Design review of the part built by this model. Coordinates are the model's own, in mm. A direction names the side the tool comes from. Give positions to 0.01 mm unless a question says otherwise; leave off trailing zeros. Write each loop counter-clockwise with the first axis right and the second up, starting at its lowest first coordinate (ties: lowest second). Pieces come first, ordered by that corner, then holes. Notation, with made-up numbers: (53.5, 66) - (108.5, 66) arc R17 ccw to (108.5, 73) - close; hole circle Ø5 at (87, 9). An arc over 180 degrees is marked (long way). Use a Markdown table: item, result. Add a question column.
```python
from build123d import *

# Parameters (mm, degrees)
BASE_DEPTH                = 38.1
DOVETAIL_CUTS_DEPTH       = 30.48
SKETCH3_R                 = 31.115
LOWER_WASHER_LIP_DEPTH    = 0.8128
SKETCH4_R                 = 44.069
SKETCH4_R_2               = 41.529
RETAINING_LIP_DEPTH       = 1.8288
SKETCH6_R                 = 30.48
UPPER_BEARING_LIP_DEPTH   = 2.797175
SKETCH7_R                 = 22.225
CENTRAL_SHAFT_DEPTH       = 26.67
SKETCH5_R                 = 7.62
NUT_CLEARANCE_SHAFT_DEPTH = 44.45
SKETCH8_R                 = 10.795
THROUGH_SHAFT_DEPTH       = 14.7574
SKETCH9_R                 = 4.1275
THROUGH_HOLE_DEPTH        = 108.091797456
NUT_SLOT_DEPTH            = 5.6007
UPPER_START               = -1.016
SKETCH11_R                = 10.795
SKETCH11_R_2              = 9.398
UPPER_WASHER_LIP_DEPTH    = 1.016
FILLET2_R                 = 50.8


with BuildPart() as part:
    # Sketch1 → Base (new body)
    with BuildSketch(Plane(origin=(0, 0, 0), x_dir=(1, 0, 0), z_dir=(0, 1, 0))):
        Polygon((-47.732745366, -19.7715505), (-47.732745366, 19.7715505), (-31.058071097, 31.058071097), (-19.7715505, 47.732745366), (19.7715505, 47.732745366), (31.058071097, 31.058071097), (47.732745366, 19.7715505), (47.732745366, -19.7715505), (31.058071097, -31.058071097), (19.7715505, -47.732745366), (-19.7715505, -47.732745366), (-31.058071097, -31.058071097), align=None)
    extrude(amount=BASE_DEPTH)

    # Sketch2 → Dovetail cuts (cut)
    with BuildSketch(Plane.XZ):
        Polygon((6.055553628, -47.732745366), (-6.055553628, -47.732745366), (-11.43, -17.252745366), (11.43, -17.252745366), align=None)
        Polygon((-17.252745366, -11.43), (-17.252745366, 11.43), (-47.732745366, 6.055553628), (-47.732745366, -6.055553628), align=None)
        Polygon((17.252745366, 11.43), (17.252745366, -11.43), (47.732745366, -6.055553628), (47.732745366, 6.055553628), align=None)
        Polygon((6.055553628, 47.732745366), (11.43, 17.252745366), (-11.43, 17.252745366), (-6.055553628, 47.732745366), align=None)
    extrude(amount=-DOVETAIL_CUTS_DEPTH, mode=Mode.SUBTRACT)

    # Sketch3 → Lower washer lip (add)
    with BuildSketch(Plane(origin=(0, 38.1, 0), x_dir=(1, 0, 0), z_dir=(0, 1, 0))):
        with Locations(Location((0, 0, 0), (0, 0, 270))):
            Circle(SKETCH3_R)
    extrude(amount=LOWER_WASHER_LIP_DEPTH)

    # Sketch4 → Retaining lip (add)
    with BuildSketch(Plane(origin=(0, 38.1, 0), x_dir=(1, 0, 0), z_dir=(0, 1, 0))):
        with Locations(Location((0, 0, 0), (0, 0, 45.946261879))):
            Circle(SKETCH4_R)
        with Locations(Location((0, 0, 0), (0, 0, 270))):
            Circle(SKETCH4_R_2, mode=Mode.SUBTRACT)
    extrude(amount=RETAINING_LIP_DEPTH)

    # Sketch6 → Upper bearing lip (add)
    with BuildSketch(Plane(origin=(0, 38.9128, 0), x_dir=(1, 0, 0), z_dir=(0, 1, 0))):
        with Locations(Location((0, 0, 0), (0, 0, 270))):
            Circle(SKETCH6_R)
    extrude(amount=UPPER_BEARING_LIP_DEPTH)

    # Sketch7 → Central shaft (add)
    with BuildSketch(Plane(origin=(0, 41.709975, 0), x_dir=(1, 0, 0), z_dir=(0, 1, 0))):
        with Locations(Location((0, 0, 0), (0, 0, 270))):
            Circle(SKETCH7_R)
    extrude(amount=CENTRAL_SHAFT_DEPTH)

    # Sketch5 → Nut clearance shaft (cut)
    with BuildSketch(Plane.XZ):
        with Locations(Location((0, 0, 0), (0, 0, 270))):
            Circle(SKETCH5_R)
    extrude(amount=-NUT_CLEARANCE_SHAFT_DEPTH, mode=Mode.SUBTRACT)

    # Sketch8 → Through Shaft (add)
    with BuildSketch(Plane(origin=(0, 68.379975, 0), x_dir=(1, 0, 0), z_dir=(0, 1, 0))):
        with Locations(Location((0, 0, 0), (0, 0, 90))):
            Circle(SKETCH8_R)
    extrude(amount=THROUGH_SHAFT_DEPTH)

    # Sketch9 → Through Hole (cut, through all)
    with BuildSketch(Plane(origin=(0, 83.137375, 0), x_dir=(1, 0, 0), z_dir=(0, 1, 0))):
        with Locations(Location((0, 0, 0), (0, 0, 270))):
            Circle(SKETCH9_R)
    extrude(amount=-THROUGH_HOLE_DEPTH, mode=Mode.SUBTRACT)

    # Sketch10 → Nut slot (cut)
    with BuildSketch(Plane.XZ.offset(-44.45)):
        Polygon((3.287458414, 5.694045), (6.574916827, 0), (3.287458414, -5.694045), (-3.287458414, -5.694045), (-6.574916827, 0), (-3.287458414, 5.694045), align=None)
    extrude(amount=-NUT_SLOT_DEPTH, mode=Mode.SUBTRACT)

    # Sketch11 → Upper washer lip (cut)
    with BuildSketch(Plane(origin=(0, 83.137375, 0), x_dir=(1, 0, 0), z_dir=(0, 1, 0)).offset(UPPER_START)):
        with Locations(Location((0, 0, 0), (0, 0, 90))):
            Circle(SKETCH11_R)
        with Locations(Location((0, 0, 0), (0, 0, 270))):
            Circle(SKETCH11_R_2, mode=Mode.SUBTRACT)
    extrude(amount=UPPER_WASHER_LIP_DEPTH, mode=Mode.SUBTRACT)

    # Fillet2
    # the kernel refuses this fillet: 50.8 mm, written as the material it adds along each edge
    with BuildSketch(Plane(origin=(-31.058071097, 0, 31.058071097), x_dir=(-0.8281314013708309, 0, -0.5605340150816753), z_dir=(0, 1, 0)), Plane(origin=(31.058071097, 0, 31.058071097), x_dir=(-0.5605340150816742, 0, 0.8281314013708316), z_dir=(0, 1, 0))) as fillet2_piece_1:
        with BuildLine():
            CenterArc((FILLET2_R * 0.192701123769, FILLET2_R), FILLET2_R, 248.185472983, 21.814527017)
            Line((-FILLET2_R * 0.178902112104, FILLET2_R * 0.0716083611488), (0, 0))
            Line((0, 0), (FILLET2_R * 0.192701123769, 0))
        make_face()
    extrude(amount=38.1)
    with BuildSketch(Plane(origin=(-31.058071097, 0, -31.058071097), x_dir=(-0.8281314013708309, 0, 0.5605340150816753), z_dir=(0, 1, 0)), Plane(origin=(31.058071097, 0, -31.058071097), x_dir=(-0.5605340150816742, 0, -0.8281314013708316), z_dir=(0, 1, 0))) as fillet2_piece_2:
        with BuildLine():
            CenterArc((FILLET2_R * 0.192701123769, -FILLET2_R), FILLET2_R, 90, 21.814527017)
            Line((-FILLET2_R * 0.178902112104, -FILLET2_R * 0.0716083611488), (0, 0))
            Line((0, 0), (FILLET2_R * 0.192701123769, 0))
        make_face()
    extrude(amount=38.1)


solid = part.part
```
(1) Mouldability with a two-part tool opening along Z and no side actions: class faces 1 (the face through (-22.4, 41.71, 2.1)), 2 (the face through (0, 30.48, 33)), 3 (the face through (-22.63, 18.78, 43.51)), 4 (the face through (-31.815, 18.783, -31.623)) as +Z half, -Z half, draft (parallel to the pull), parting line (faces both ways), or undercut.
(2) For line 1 along Z through (x, y) = (-0.5, 12); line 2 along X through (y, z) = (38, 0); line 3 along X through (y, z) = (63.5, 0) (1 decimal), list the stretches that pass through material, from the lowest coordinate up.
(3) Tool access review of faces 5 (the face through (0, 30.48, -32)), 6 (the face through (9.346, 38.501, 29.678)), 7 (the face through (22.71, 18.78, 43.39)): name each direction out of +Z, -Z, +X, -X, +Y, -Y from which nothing blocks a thin tool from reaching the whole face with its end or side.
(4) Add section D-D (z = -15.5). State the section outline as (x, y) points.
(5) Insertion check: pin 1 (1 mm diameter, centred on x = -0.5, y = 40, fed in from -Z); pin 2 (1 mm diameter, centred on x = -19.5, z = 5.5, fed in from -Y); pin 3 (5 mm diameter, centred on x = -14, z = 35, fed in from +Y). Each pin has a flat end and moves straight along its axis. Give the tip position at first contact, or say it passes through.
(6) Add section C-C (z = 37.5). State the section outline as (x, y) points, and give its area (3 significant figures).
(7) Add section B-B (x = 35.5). State the section outline as (y, z) points.
Answers follow:
| question | item | result |
|---|---|---|
| 1 | face 1 | draft |
| 1 | face 2 | undercut |
| 1 | face 3 | +Z half |
| 1 | face 4 | -Z half |
| 2 | line 1 | -17.25 to -7.6, 7.6 to 17.25 |
| 2 | line 2 | -47.73 to -7.62, 7.62 to 47.73 |
| 2 | line 3 | -22.2 to -4.1, 4.1 to 22.2 |
| 3 | face 5 | -Y |
| 3 | face 6 | +Y |
| 3 | face 7 | +Z, +X, +Y, -Y |
| 4 | outline | (-47.73, 0) - (47.73, 0) - (47.73, 38.1) - (41.25, 38.1) - (41.25, 39.93) - (38.53, 39.93) - (38.53, 38.1) - (26.98, 38.1) - (26.98, 38.91) - (26.24, 38.91) - (26.24, 41.71) - (15.93, 41.71) - (15.93, 68.38) - (-15.93, 68.38) - (-15.93, 41.71) - (-26.24, 41.71) - (-26.24, 38.91) - (-26.98, 38.91) - (-26.98, 38.1) - (-38.53, 38.1) - (-38.53, 39.93) - (-41.25, 39.93) - (-41.25, 38.1) - (-47.73, 38.1) - close |
| 5 | pin 1 | z = -44.07 |
| 5 | pin 2 | y = 30.48 |
| 5 | pin 3 | y = 38.1 |
| 6 | outline | (-26.75, 0) - (-7.86, 0) - (-7.86, 30.48) - (7.86, 30.48) - (7.86, 0) - (26.75, 0) - (26.75, 38.1) - (23.15, 38.1) - (23.15, 39.93) - (17.84, 39.93) - (17.84, 38.1) - (-17.84, 38.1) - (-17.84, 39.93) - (-23.15, 39.93) - (-23.15, 38.1) - (-26.75, 38.1) - close |
| 6 | area | 1,580 mm^2 |
| 7 | outline | (0, -28.3) - (38.1, -28.3) - (38.1, -26.11) - (39.93, -26.11) - (39.93, -21.55) - (38.1, -21.55) - (38.1, 21.55) - (39.93, 21.55) - (39.93, 26.11) - (38.1, 26.11) - (38.1, 28.3) - (0, 28.3) - (0, 8.21) - (30.48, 8.21) - (30.48, -8.21) - (0, -8.21) - close |
